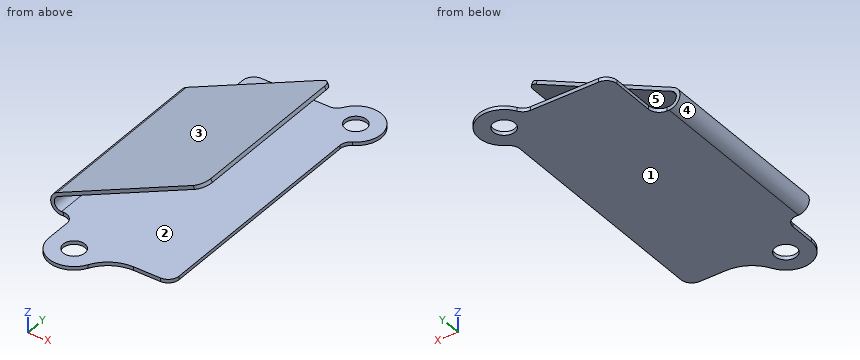
```python
from build123d import *

# Parameters (mm, degrees)
SKETCH1_R           = 3
BOSS_EXTRUDE1_DEPTH = 1
EDGE_FLANGE1_DEPTH  = 50
FILLET1_R           = 3
FILLET2_R           = 10


# Sheet-metal steps are written as plain solids
with BuildPart() as part:
    # Sketch1 → Boss-Extrude1 (new body)
    with BuildSketch(Plane.XY):
        with BuildLine():
            Line((6.708203932, 2), (25.4, 2))
            Line((25.4, 2), (25.4, 69.262789895))
            ThreePointArc((25.4, 69.262789895), (28.486423204, 80.912797943), (16.791796068, 78))
            Line((16.791796068, 78), (-7, 78))
            Line((-7, 78), (-7, 60))
            Line((-7, 60), (-10.6, 60))
            Line((-10.6, 60), (-10.6, 10))
            Line((-10.6, 10), (-7, 10))
            Line((-7, 10), (-7, 0))
            ThreePointArc((-7, 0), (1.010587075, -6.926666858), (6.708203932, 2))
        make_face()
        Circle(SKETCH1_R, mode=Mode.SUBTRACT)
        with Locations((23.5, 76)):
            Circle(SKETCH1_R, mode=Mode.SUBTRACT)
    extrude(amount=BOSS_EXTRUDE1_DEPTH)

    # Edge-Flange1 section (across the edge) → Edge-Flange1 (add)
    with BuildSketch(Plane(origin=(-19.621417007, 60, 1), x_dir=(0.4226182617407006, 0, -0.9063077870366494), z_dir=(0, -1, 0))):
        with BuildLine():
            Line((-1, 9.021417007), (-1, 53.489291496))
            Line((-1, 53.489291496), (0, 53.489291496))
            Line((0, 53.489291496), (0, 9.021417007))
            ThreePointArc((0, 9.021417007), (1.567120772, 7.068824993), (3.812615574, 8.176180484))
            Line((3.812615574, 8.176180484), (4.718923361, 7.753562222))
            ThreePointArc((4.718923361, 7.753562222), (1.350681158, 6.092528986), (-1, 9.021417007))
        make_face()
    extrude(amount=EDGE_FLANGE1_DEPTH)

    # Fillet1
    fillet1_edges = [part.edges().sort_by_distance(p)[0] for p in [
        (-7, 78, 0.5),
        (-7, 60, 0.5),
        (-7, 10, 0.5),
        (25.4, 2, 0.5),
        (25.4, 69.262789895, 0.5),
        (16.791796068, 78, 0.5),
        (28.645035268, 60, 24.058705287),
        (28.645035268, 10, 24.058705287),
    ]]
    fillet(fillet1_edges, radius=FILLET1_R)

    # Fillet2
    fillet2_edges = [part.edges().sort_by_distance(p)[0] for p in [
        (6.708203932, 2, 0.5),
    ]]
    fillet(fillet2_edges, radius=FILLET2_R)


solid = part.part
```
For this review, take the finished solid that the model builds, in its own axes (mm). Face numbers are marked on the shaded views. A direction names the side the tool comes from. Round coordinates to 2 decimals unless told otherwise and drop trailing zeros. Write each loop counter-clockwise with the first axis right and the second up, starting at its lowest first coordinate (ties: lowest second). Pieces come first, ordered by that corner, then holes.
1) Insertion check: pin 1 Ø11.5 at (x, z) = (10.5, 8.5) entering from +Y; pin 2 Ø6 at (x, y) = (15, 10) entering from -Z; pin 3 Ø0.5 at (y, z) = (2.5, 0.5) entering from -X; pin 4 Ø1.5 at (y, z) = (53, 8) entering from -X. Each pin has a flat end and moves straight along its axis. Give the tip position at first contact, or say it passes through.
Answer below:
pin 1: passes through
pin 2: stops at z = 0
pin 3: stops at x = -7
pin 4: stops at x = -8.58
2) Mouldability with a two-part tool opening along Z and no side actions: class the marked faces 3, 4 and 5 as +Z half, -Z half, draft (parallel to the pull), parting line (faces both ways), or undercut.
Answer below:
face 3: +Z half
face 4: parting line
face 5: undercut
3) Take a section at D-D on x = 9. Give the boundary of the cut face in (y, z).
Answer below:
outline: (0, 0) - (78, 0) - (78, 1) - (0, 1) - close; (10, 14.35) - (60, 14.35) - (60, 15.45) - (10, 15.45) - close
4) Take a section at A-A on x = 0. Give the boundary of the cut face in (y, z).
Answer below:
outline: (-7, 0) - (-3, 0) - (-3, 1) - (-7, 1) - close; (3, 0) - (78, 0) - (78, 1) - (3, 1) - close; (10, 10.15) - (60, 10.15) - (60, 11.25) - (10, 11.25) - close
5) Machinability: for the marked faces 1 and 2, which of the approach directions +Z, -Z, +X, -X, +Y, -Y give a long, thin tool a straight path to every point of the face, cutting with its end or side? Answer none if there is none.
Answer below:
face 1: -Z, +X, -X, +Y, -Y
face 2: +X, +Y, -Y
6) Take a section at C-C on y = 55. Give the boundary of the cut face in (x, z), then the cut area to 3 significant figures.
Answer below:
outline: (-11.87, 5.72) arc R3 ccw to (-10.6, 0) - (25.4, 0) - (25.4, 1) - (-10.6, 1) arc R2 cw to (-11.45, 4.81) - (28.86, 23.61) - (28.43, 24.51) - close
area: 87.2 mm2
7) Take a section at B-B on y = 76. Give the boundary of the cut face in (x, z).
Answer below:
outline: (-6.83, 0) - (20.5, 0) - (20.5, 1) - (-6.83, 1) - close; (26.5, 0) - (30.5, 0) - (30.5, 1) - (26.5, 1) - close
8) For line 1 along Y through (x, z) = (0, 0.4); line 2 along Z through (x, y) = (5.5, 41); line 3 along Z through (x, y) = (4, 76.5), list the stretches that pass through material, from the lowest coordinate up.
Answer below:
line 1: y = -7 to -3, 3 to 78
line 2: z = 0 to 1, 12.71 to 13.82
line 3: z = 0 to 1
